Part model, mm, in its own coordinate system. A direction names the side the tool comes from. Round coordinates to 2 decimals unless told otherwise and drop trailing zeros. Loops run counter-clockwise (first coordinate to the right, second up) from the corner with the lowest first, then second, coordinate; pieces in that order, holes last. Notation, with made-up numbers: (2, -38) -> (35, -38) arc R13 cw to (35, -30) -> close; hole circle Ø4 at (-17, -18.75). An arc over 180 degrees is marked (long way). Use a Markdown table: item, result. Add a question column.
Item 1: Which spindle directions (+Z, -Z, +X, -X, +Y, -Y) get a long thin tool onto all of the face, cutting with end or side? Do faces 4 (the face through (-6.194, 0.243, -0.695)), 5 (the face through (2.83, 0.24, 3.1)), 6 (the face through (6.444, 0.243, 3.823)). Say none if no direction does.
Item 2: Probe line 1 (Z direction, x = -2, y = 0.35); line 2 (X direction, y = 0.35, z = -0.5); line 3 (Z direction, x = -3, y = 0.25). List the from-to ranges inside material, lowest first. Write a range as [from, to].
Item 3: Cut at D-D, the plane x = -6. List the corners of the cut face in (y, z).
Item 4: Cut at A-A, the plane z = -1.25. List the corners of the cut face in (x, y), plus the area to 3 significant figures.
Item 5: Cut at B-B, the plane x = 4.5. List the corners of the cut face in (y, z).
Item 6: Cut at C-C, the plane z = -4. List the corners of the cut face in (x, y), plus the area to 3 significant figures.
Item 7: Two-plate mould, pull along Z, no slides. Class faces 1 (the face through (0.089, 0.243, -7.492)), 2 (the face through (-6.533, 0.243, 3.669)), 3 (the face through (-4.1, 0.2, 0.9)): pulls with the +Z half, pulls with the -Z half, needs draft (parallel to the pull), parting line crosses it, or undercut.
```python
from build123d import *

# Parameters (mm, degrees)
SKETCH1_R           = 2.4003
BOSS_EXTRUDE1_DEPTH = 0.493268
CIRPATTERN1_COUNT   = 3
SKETCH2_R           = 1.0033
CUT_EXTRUDE3_DEPTH  = 11.608176626
CIRPATTERN2_COUNT   = 3
FILLET1_R           = 2.54


with BuildPart() as part:
    # Sketch1 → Boss-Extrude1 (new body)
    with BuildSketch(Plane(origin=(0, 0, 0), x_dir=(1, 0, 0), z_dir=(0, 1, 0))):
        with BuildLine():
            ThreePointArc((-2.080029721, 5.48099038), (-1.52284746, 5.377722752), (-1.27, 4.870589203))
            Line((-1.27, 4.870589203), (-1.27, 2.036796526))
            ThreePointArc((-1.27, 2.036796526), (0, 2.4003), (1.27, 2.036796526))
            Line((1.27, 2.036796526), (1.27, 4.870589203))
            ThreePointArc((1.27, 4.870589203), (1.52284746, 5.377722752), (2.080029721, 5.48099038))
            Line((2.080029721, 5.48099038), (5.363123917, 4.539578268))
            ThreePointArc((5.363123917, 4.539578268), (5.647788598, 4.647944118), (5.62377215, 4.951589221))
            ThreePointArc((5.62377215, 4.951589221), (0, 7.493), (-5.62377215, 4.951589221))
            ThreePointArc((-5.62377215, 4.951589221), (-5.647788598, 4.647944118), (-5.363123917, 4.539578268))
            Line((-5.363123917, 4.539578268), (-2.080029721, 5.48099038))
        make_face()
        Circle(SKETCH1_R)
    boss_extrude1 = extrude(amount=BOSS_EXTRUDE1_DEPTH)

    # CirPattern1: Boss-Extrude1 ×3 about axis
    cirpattern1_axis = Axis((0, 0, 0), (0, 1, 0))
    for i in range(1, CIRPATTERN1_COUNT):
        add(boss_extrude1.rotate(cirpattern1_axis, i * 360 / CIRPATTERN1_COUNT))

    # Sketch2 → Cut-Extrude3 (cut, through all)
    with BuildSketch(Plane(origin=(0, 0.493268, 0), x_dir=(1, 0, 0), z_dir=(0, 1, 0))):
        Circle(SKETCH2_R)
        with BuildLine():
            Line((0.3175, 0.951737695), (0.3175, 1.5367))
            Line((0.3175, 1.5367), (-0.3175, 1.5367))
            Line((-0.3175, 1.5367), (-0.3175, 0.951737695))
            ThreePointArc((-0.3175, 0.951737695), (0, 1.0033), (0.3175, 0.951737695))
        make_face()
    cut_extrude3 = extrude(amount=-CUT_EXTRUDE3_DEPTH, mode=Mode.SUBTRACT)

    # CirPattern2: Cut-Extrude3 ×3 about axis
    cirpattern2_axis = Axis((0, 0, 0), (0, 1, 0))
    for i in range(1, CIRPATTERN2_COUNT):
        add(cut_extrude3.rotate(cirpattern2_axis, i * 360 / CIRPATTERN2_COUNT), mode=Mode.SUBTRACT)

    # Fillet1
    fillet1_edges = [part.edges().sort_by_distance(p)[0] for p in [
        (1.27, 0.246634, -2.036796526),
        (-1.27, 0.246634, -2.036796526),
        (2.398917534, 0.246634, -0.081454),
        (-1.128917534, 0.246634, 2.118250526),
        (-2.398917534, 0.246634, -0.081454),
        (1.128917534, 0.246634, 2.118250526),
    ]]
    fillet(fillet1_edges, radius=FILLET1_R)


solid = part.part
```
A:
| question | item | result |
|---|---|---|
| 1 | face 4 | -Z, +Y, -Y |
| 1 | face 5 | +Y, -Y |
| 1 | face 6 | +X, +Y, -Y |
| 2 | line 1 | z = [-7.22, -5.5], [-1.33, 2.62], [6.19, 7.22] |
| 2 | line 2 | x = [-7.48, -6.15], [-2.4, -0.87], [0.87, 2.4], [6.15, 7.48] |
| 2 | line 3 | z = [-6.87, -5.22], [0.22, 3.2], [5.22, 6.87] |
| 3 | outline | (0, 0.08) -> (0.49, 0.08) -> (0.49, 4.49) -> (0, 4.49) -> close |
| 4 | outline | (-7.39, 0) -> (-6.33, 0) -> (-6.33, 0.49) -> (-7.39, 0.49) -> close; (-2.05, 0) -> (-0.32, 0) -> (-0.32, 0.49) -> (-2.05, 0.49) -> close; (0.32, 0) -> (2.05, 0) -> (2.05, 0.49) -> (0.32, 0.49) -> close; (6.33, 0) -> (7.39, 0) -> (7.39, 0.49) -> (6.33, 0.49) -> close |
| 4 | area | 2.75 mm^2 |
| 5 | outline | (0, -5.99) -> (0.49, -5.99) -> (0.49, -4.79) -> (0, -4.79) -> close; (0, 1.13) -> (0.49, 1.13) -> (0.49, 5.99) -> (0, 5.99) -> close |
| 6 | outline | (-1.27, 0) -> (1.27, 0) -> (1.27, 0.49) -> (-1.27, 0.49) -> close |
| 6 | area | 1.25 mm^2 |
| 7 | face 1 | pulls with the -Z half |
| 7 | face 2 | parting line crosses it |
| 7 | face 3 | undercut |
